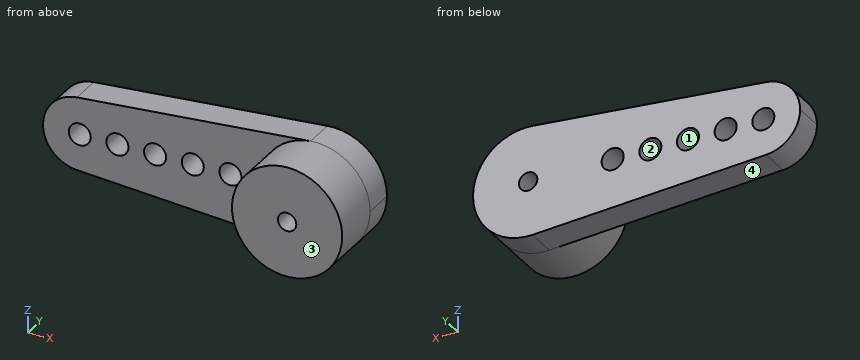
from build123d import *

# Parameters (mm, degrees)
BOSS_EXTRUDE1_DEPTH = 1.7
SKETCH2_R           = 0.6
CUT_EXTRUDE1_DEPTH  = 2.7
SKETCH3_R           = 3
BOSS_EXTRUDE2_DEPTH = 2.8
SKETCH4_R           = 0.5
CUT_EXTRUDE2_DEPTH  = 5.5


with BuildPart() as part:
    # Sketch1 → Boss-Extrude1 (new body)
    with BuildSketch(Plane(origin=(0, 0, 0), x_dir=(1, 0, 0), z_dir=(0, 1, 0))):
        with BuildLine():
            Line((-3, 0), (-10.8, 0))
            ThreePointArc((-10.8, 0), (-11.442152439, -1.468417516), (-12.95625, -1.993887143))
            Line((-12.95625, -1.993887143), (-0.234375, -2.990830714))
            ThreePointArc((-0.234375, -2.990830714), (-2.202626273, -2.036771342), (-3, 0))
        make_face()
        with BuildLine():
            ThreePointArc((-12.95625, 1.993887143), (-14.268417516, 1.357847561), (-14.8, 0))
            Line((-14.8, 0), (-10.8, 0))
            ThreePointArc((-10.8, 0), (-11.442152439, 1.468417516), (-12.95625, 1.993887143))
        make_face()
        with BuildLine():
            Line((-10.8, 0), (-14.8, 0))
            ThreePointArc((-14.8, 0), (-14.268417516, -1.357847561), (-12.95625, -1.993887143))
            ThreePointArc((-12.95625, -1.993887143), (-11.442152439, -1.468417516), (-10.8, 0))
        make_face()
        with BuildLine():
            ThreePointArc((-12.95625, 1.993887143), (-11.442152439, 1.468417516), (-10.8, 0))
            Line((-10.8, 0), (-3, 0))
            ThreePointArc((-3, 0), (-2.202626273, 2.036771342), (-0.234375, 2.990830714))
            Line((-0.234375, 2.990830714), (-12.95625, 1.993887143))
        make_face()
        with BuildLine():
            ThreePointArc((-0.234375, 2.990830714), (-2.202626273, 2.036771342), (-3, 0))
            Line((-3, 0), (3, 0))
            ThreePointArc((3, 0), (2.036771342, 2.202626273), (-0.234375, 2.990830714))
        make_face()
        with BuildLine():
            Line((3, 0), (-3, 0))
            ThreePointArc((-3, 0), (-2.202626273, -2.036771342), (-0.234375, -2.990830714))
            ThreePointArc((-0.234375, -2.990830714), (2.036771342, -2.202626273), (3, 0))
        make_face()
    extrude(amount=BOSS_EXTRUDE1_DEPTH)

    # Sketch2 → Cut-Extrude1 (cut, through all)
    with BuildSketch(Plane(origin=(0, 1.7, 0), x_dir=(1, 0, 0), z_dir=(0, 1, 0))):
        with Locations((-12.8, 0)):
            Circle(SKETCH2_R)
        with Locations((-10.75, 0)):
            Circle(SKETCH2_R)
        with Locations((-8.7, 0)):
            Circle(SKETCH2_R)
        with Locations((-6.65, 0)):
            Circle(SKETCH2_R)
        with Locations((-4.6, 0)):
            Circle(SKETCH2_R)
    extrude(amount=-CUT_EXTRUDE1_DEPTH, mode=Mode.SUBTRACT)

    # Sketch3 → Boss-Extrude2 (add)
    with BuildSketch(Plane.XZ):
        Circle(SKETCH3_R)
    extrude(amount=BOSS_EXTRUDE2_DEPTH)

    # Sketch4 → Cut-Extrude2 (cut, through all)
    with BuildSketch(Plane.XZ.offset(2.8)):
        Circle(SKETCH4_R)
    extrude(amount=-CUT_EXTRUDE2_DEPTH, mode=Mode.SUBTRACT)


solid = part.part
Verification items for the finished model (mm, model axes). Face numbers are marked on the shaded views. Round coordinates to 2 decimals unless told otherwise and drop trailing zeros. Loops run counter-clockwise (first coordinate to the right, second up) from the corner with the lowest first, then second, coordinate; pieces in that order, holes last. Notation, with made-up numbers: (42.5, 1.25) - (93.5, 1.25) arc R20 ccw to (93.5, 37.25) - close; hole circle Ø5 at (-29.75, 31). An arc over 180 degrees is marked (long way). Answer in a Markdown table with one row per item. Add a question column.
Q1. Release check for a two-part mould opening along Z. For the marked faces 1, 2, 3 and 4 record: pulls with the +Z half, pulls with the -Z half, needs draft (parallel to the pull), parting line crosses it, or undercut.
Q2. Section check B-B on y = 0.7. Enter the section's corners in (x, z).
Q3. Gauge pin test, flat ends, axial feed: pin 1 (1.4 mm diameter, centred on x = -8.7, z = 0, fed in from -Y); pin 2 (1 mm diameter, centred on y = 1, z = -1.5, fed in from +X). Record the tip position at first contact, or that the pin passes through.
Q4. Section check A-A on x = 0. Enter the section's corners in (y, z).
Q5. Material ranges on line 1 (Z direction, x = 0, y = 0.75); line 2 (Z direction, x = -10.75, y = 0.6); line 3 (Y direction, x = -11, z = 1), recorded low to high.
Q6. Section check D-D on x = -6.65. Enter the section's corners in (y, z), plus the area to 3 significant figures.
Q7. Section check C-C on z = 2.25. Enter the section's corners in (x, y), plus the area to 3 significant figures.
Found:
| question | item | result |
|---|---|---|
| 1 | face 1 | undercut |
| 1 | face 2 | undercut |
| 1 | face 3 | needs draft |
| 1 | face 4 | pulls with the -Z half |
| 2 | outline | (-12.96, -1.99) - (-0.23, -2.99) arc R3 ccw (long way) to (-0.23, 2.99) - (-12.96, 1.99) arc R2 ccw to start; hole circle Ø1.2 at (-12.8, 0); hole circle Ø1.2 at (-10.75, 0); hole circle Ø1.2 at (-8.7, 0); hole circle Ø1.2 at (-6.65, 0); hole circle Ø1.2 at (-4.6, 0); hole circle Ø1 at (0, 0) |
| 3 | pin 1 | stops at y = 0 |
| 3 | pin 2 | stops at x = 2.83 |
| 4 | outline | (-2.8, -3) - (1.7, -3) - (1.7, -0.5) - (-2.8, -0.5) - close; (-2.8, 0.5) - (1.7, 0.5) - (1.7, 3) - (-2.8, 3) - close |
| 5 | line 1 | z = -3 to -0.5, 0.5 to 3 |
| 5 | line 2 | z = -2.17 to -0.6, 0.6 to 2.17 |
| 5 | line 3 | y = 0 to 1.7 |
| 6 | outline | (0, -2.49) - (1.7, -2.49) - (1.7, -0.6) - (0, -0.6) - close; (0, 0.6) - (1.7, 0.6) - (1.7, 2.49) - (0, 2.49) - close |
| 6 | area | 6.42 mm² |
| 7 | outline | (-9.69, 0) - (-1.98, 0) - (-1.98, -2.8) - (1.98, -2.8) - (1.98, 1.7) - (-9.69, 1.7) - close |
| 7 | area | 31.0 mm² |
